Build history of the part. All positions in model axes, mm. Face numbers are marked on the shaded views. A direction names the side the tool comes from. Give positions to 0.01 mm unless a question says otherwise; leave off trailing zeros. Order: outer loops, then holes, each group sorted by start corner. A loop starts at its lowest first (then second) coordinate and runs counter-clockwise, first axis right, second up. Notation, with made-up numbers: (89.5, 12) - (114.5, 12) arc R29 cw to (114.5, 44) - close; hole circle Ø10 at (-17.5, 48). An arc over 180 degrees is marked (long way). One line per item, written item: value.
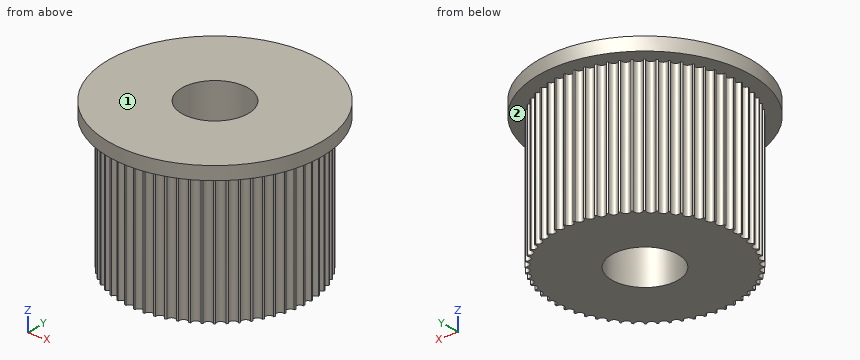
```python
from build123d import *

# Parameters (mm, degrees)
SKETCH1_R           = 7
BOSS_EXTRUDE1_DEPTH = 10
SKETCH2_R           = 8
BOSS_EXTRUDE2_DEPTH = 1
SKETCH3_R           = 2.5
CUT_EXTRUDE1_DEPTH  = 17
SKETCH4_R           = 0.3
CUT_EXTRUDE2_DEPTH  = 10
CIRPATTERN1_COUNT   = 60


with BuildPart() as part:
    # Sketch1 → Boss-Extrude1 (new body)
    with BuildSketch(Plane.XY):
        Circle(SKETCH1_R)
    extrude(amount=BOSS_EXTRUDE1_DEPTH)

    # Sketch2 → Boss-Extrude2 (add)
    with BuildSketch(Plane.XY.offset(10)):
        Circle(SKETCH2_R)
    extrude(amount=BOSS_EXTRUDE2_DEPTH)

    # Sketch3 → Cut-Extrude1 (cut)
    with BuildSketch(Plane(origin=(0, 0, 0), x_dir=(-1, 0, 0), z_dir=(0, 0, -1))):
        Circle(SKETCH3_R)
    extrude(amount=-CUT_EXTRUDE1_DEPTH, mode=Mode.SUBTRACT)

    # Sketch4 → Cut-Extrude2 (cut)
    with BuildSketch(Plane(origin=(0, 0, 0), x_dir=(-1, 0, 0), z_dir=(0, 0, -1))):
        with Locations((0, 7)):
            Circle(SKETCH4_R)
    cut_extrude2 = extrude(amount=-CUT_EXTRUDE2_DEPTH, mode=Mode.SUBTRACT)

    # CirPattern1: Cut-Extrude2 ×60 about axis
    cirpattern1_axis = Axis((0, 0, 0), (0, 0, 1))
    for i in range(1, CIRPATTERN1_COUNT):
        add(cut_extrude2.rotate(cirpattern1_axis, i * 360 / CIRPATTERN1_COUNT), mode=Mode.SUBTRACT)


solid = part.part
```
(1) Slice it at C-C, the plane y = -3.5. Give the cut face in (x, z).
Completed:
outline: (-7.19, 10) - (-5.76, 10) - (-5.76, 0) - (5.76, 0) - (5.76, 10) - (7.19, 10) - (7.19, 11) - (-7.19, 11) - close
(2) Slice it at A-A, the plane y = 0. Give the cut face in (x, z), and give its area (3 significant figures).
Completed:
outline: (-8, 10) - (-6.7, 10) - (-6.7, 0) - (-2.5, 0) - (-2.5, 11) - (-8, 11) - close; (2.5, 0) - (6.7, 0) - (6.7, 10) - (8, 10) - (8, 11) - (2.5, 11) - close
area: 95.0 mm²
(3) 3-axis set-ups, long thin cutter, end or side, ignore diameter. For the marked faces 1 and 2: which of +Z, -Z, +X, -X, +Y, -Y reach the whole face in a straight line?
Completed:
face 1: +Z, +X, -X, +Y, -Y
face 2: -Z
(4) Pin check, flat tips, straight feed: P1, Ø2, axis at y = 0, z = 2, coming from the +X side; P2, Ø2, axis at x = 5.5, z = 3.5, coming from the +Y side; P3, Ø1.5, axis at x = 0.5, z = 7, coming from the -Y side; P4, Ø6.5, axis at x = 0, y = 0, coming from the +Z side. Stop position of each tip, or through.
Completed:
P1: x = 6.99
P2: y = 5
P3: y = -6.99
P4: z = 11
(5) Drill centre lines: line 1 (Z direction, x = -4.5, y = -5); line 2 (X direction, y = -5.25, z = 8.25); line 3 (X direction, y = 1.5, z = 9.75). Where is each one in solid material? Low to high.
Completed:
line 1: 10 to 11
line 2: -4.39 to 4.39
line 3: -6.55 to -2, 2 to 6.55
